```python
from build123d import *

# Parameters (mm, degrees)
F0_W     = 38.1
F0_H     = 88.9
F1_DEPTH = 381
F3_DEPTH = 38.101
F4_R     = 5.08
F6_D     = 6.35


# Not quite as in the source:
# - a feature names something its author has since deleted; it is built from what else it names


with BuildPart() as f1:
    # F0 (on Top) → F1 (new body, symmetric)
    with BuildSketch(Plane.XY):
        Rectangle(F0_W, F0_H)
    extrude(amount=F1_DEPTH, both=True)

    # F2 (on face) → F3 (cut, through all)
    with BuildSketch(Plane.YZ.offset(19.05)):
        Polygon((-21.4409868904, -374.8347535186), (-44.45, -381), (44.45, -381), (44.45, -357.1793167929), align=None)
        Polygon((-44.45, -288.9639475615), (-44.45, -381), (-21.4409868904, -374.8347535186), align=None)
    extrude(amount=-F3_DEPTH, mode=Mode.SUBTRACT)

    # F4
    f4_edges = [f1.edges().sort_by_distance(p)[0] for p in [
        (19.05, -44.45, 46.018026),
        (-19.05, -44.45, 46.018026),
        (19.05, 44.45, 11.910342),
        (-19.05, 44.45, 11.910342),
    ]]
    fillet(f4_edges, radius=F4_R)

    # F6 (through all)
    with Locations(Plane.YZ.offset(19.05)):
        with Locations((-25.4, 355.6), (-25.4, 317.5), (-25.4, -127), (-25.4, -165.1)):
            Hole(F6_D / 2)


solid = f1.part
```
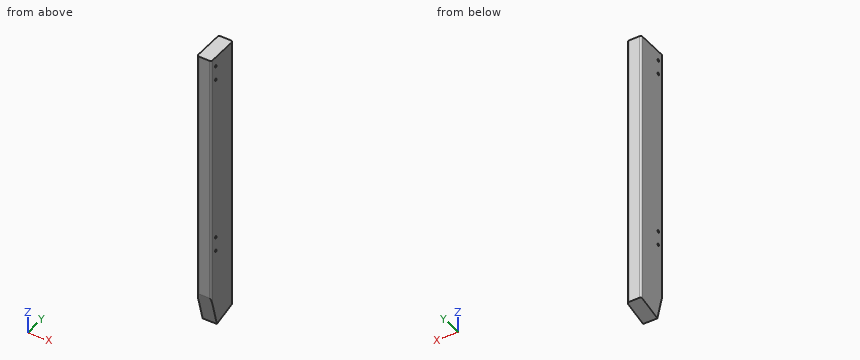
Work out the finished part from the listing and answer in its coordinate system (mm). Coordinates: 2 decimals unless noted, no trailing zeros. Loops run counter-clockwise (first coordinate to the right, second up) from the corner with the lowest first, then second, coordinate; pieces in that order, holes last. Notation, with made-up numbers: (74.25, 83.25) -> (85.25, 83.25) arc R8 cw to (85.25, 87.25) -> close; hole circle Ø4 at (27, -15.75). An arc over 180 degrees is marked (long way). Answer as CSV lines item,"result".
Q1. This flat-tipped pin is pushed along its axis until it touches: pin 1 (10 mm diameter, centred on x = 3, y = 7.5, fed in from -Z). Where does it stop, or does it pass through?
Findings:
pin 1,"stops at z = -368.42"
Q2. Find the intervals of material crossed by probe 1 along Y at (x, z) = (2, 317); probe 2 along Y at (x, z) = (4, 317.5) (3 decimals); probe 3 along Z at (x, y) = (10.5, -17), in increasing order.
Findings:
probe 1,"y = -44.45 to -28.54, -22.26 to 44.45"
probe 2,"y = -44.45 to -28.575, -22.225 to 44.45"
probe 3,"z = -373.64 to 381"
Q3. The part is cut by section A-A on x = 7. Write down the section's boundary in (y, z) (3 decimals).
Findings:
outline,"(-44.45, -288.964) -> (-21.441, -374.835) -> (44.45, -357.179) -> (44.45, 381) -> (-44.45, 381) -> close; hole circle Ø6.35 at (-25.4, -165.1); hole circle Ø6.35 at (-25.4, -127); hole circle Ø6.35 at (-25.4, 317.5); hole circle Ø6.35 at (-25.4, 355.6)"
Q4. The part is cut by section B-B on y = 23. Write down the section's boundary in (x, z), and give its area (3 significant figures).
Findings:
outline,"(-19.05, -362.93) -> (19.05, -362.93) -> (19.05, 381) -> (-19.05, 381) -> close"
area,"28,300 mm²"
